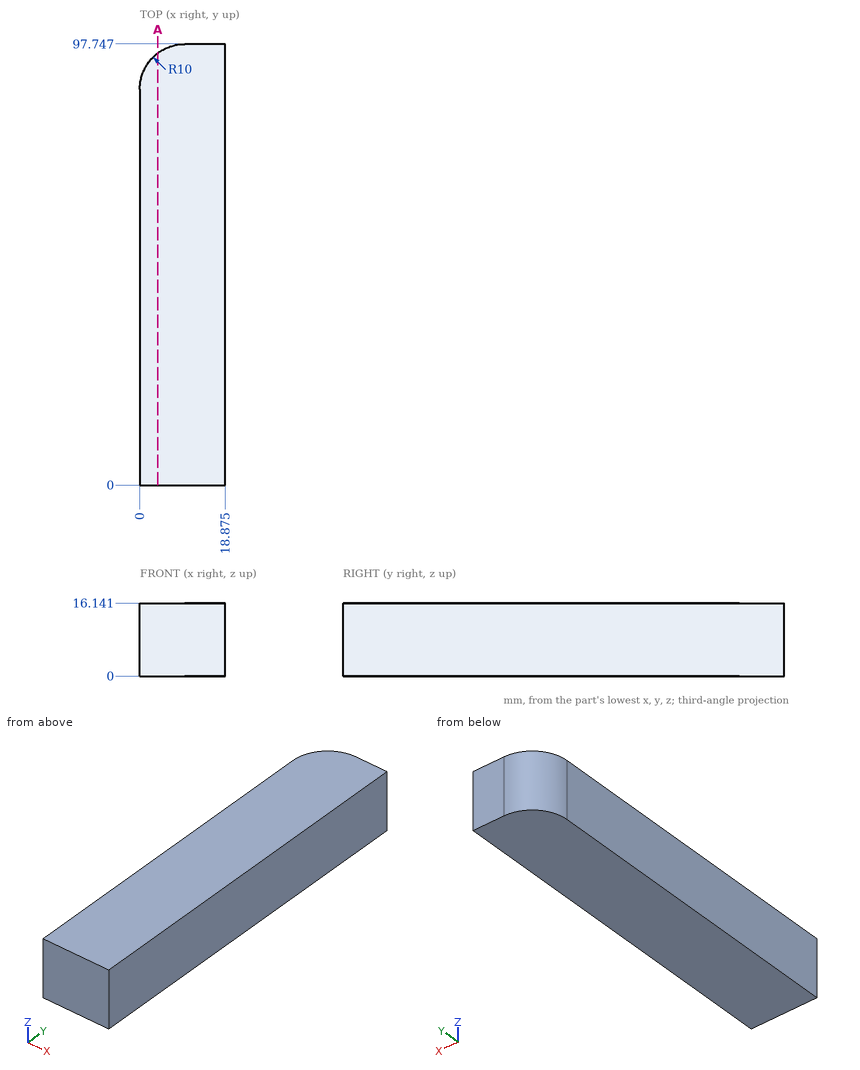
Answer from the drawing. Dimensions are ordinates in mm from the lowest x, y and z of the part. Give positions to 0.01 mm unless a question says otherwise; leave off trailing zeros. Loops run counter-clockwise (first coordinate to the right, second up) from the corner with the lowest first, then second, coordinate; pieces in that order, holes last.
Item 1: Each of these flat-tipped pins is pushed along its axis until it touches: pin 1 Ø2 at (x, y) = (16.5, 65) entering from -Z; pin 2 Ø5 at (x, z) = (3.5, 8.5) entering from +Y. Where does it stop, or does it pass through?
Derived:
pin 1: stops at z = 0
pin 2: stops at y = 96.91
Item 2: Find the intervals of material crossed by line 1 along X through (y, z) = (88, 2) (3 decimals); line 2 along Y through (x, z) = (7.75, 1.5); line 3 along X through (y, z) = (92, 8) (3 decimals), in increasing order.
Derived:
line 1: x = 0.003 to 18.875
line 2: y = 0 to 97.49
line 3: x = 0.949 to 18.875
Item 3: A cutting plane is placed at A-A (x = 4). Give the vertices of the cut face in (y, z), then the cut area to 3 significant figures.
Derived:
outline: (0, 0) - (95.75, 0) - (95.75, 16.14) - (0, 16.14) - close
area: 1,550 mm2
